Work out the finished part from the listing and answer in its coordinate system (mm). A direction names the side the tool comes from. Coordinates: 2 decimals unless noted, no trailing zeros. Loops run counter-clockwise (first coordinate to the right, second up) from the corner with the lowest first, then second, coordinate; pieces in that order, holes last. Notation, with made-up numbers: (-27.5, -7.5) -> (4.5, -7.5) arc R19 ccw to (4.5, -1.5) -> close; hole circle Ø2 at (72, 1.25). An arc over 180 degrees is marked (long way). Use a Markdown table: item, result. Add a question column.
```python
from build123d import *

# Parameters (mm, degrees)
BOSS_EXTRUDE1_DEPTH = 75
SKETCH4_W           = 56
SKETCH4_H           = 70
CUT_EXTRUDE1_DEPTH  = 36
SKETCH21_R          = 0.875
BOSS_EXTRUDE3_DEPTH = 5
CUT_EXTRUDE2_REACH  = 77
SKETCH23_W          = 11.9
SKETCH23_H          = 2.9
CUT_EXTRUDE3_REACH  = 70.5
SKETCH24_W          = 11
SKETCH24_H          = 3
CUT_EXTRUDE4_REACH  = 70.5
SKETCH25_W          = 7
SKETCH25_H          = 2
CUT_EXTRUDE5_REACH  = 70.5
SKETCH26_W          = 7.2
SKETCH26_H          = 2
CUT_EXTRUDE6_REACH  = 77
SKETCH27_W          = 16
SKETCH27_H          = 2.9
CUT_EXTRUDE7_REACH  = 70.5
SKETCH28_W          = 6
SKETCH28_H          = 9
CUT_EXTRUDE8_REACH  = 70.5
SKETCH29_W          = 21
SKETCH29_H          = 5
CUT_EXTRUDE9_REACH  = 77
SKETCH30_W          = 6
SKETCH30_H          = 8
CUT_EXTRUDE10_REACH = 70.5
SKETCH31_W          = 49
SKETCH31_H          = 7
CUT_EXTRUDE11_REACH = 70.5
SKETCH32_W          = 6
SKETCH32_H          = 7


with BuildPart() as part:
    # Sketch1 → Boss-Extrude1 (new body)
    with BuildSketch(Plane.XY):
        Polygon((-37.771390637, 7.690116692), (-37.771390637, 10.690116692), (38.228609363, 10.690116692), (38.228609363, 7.690116692), (30.728609363, 7.690116692), (30.728609363, -28.309883308), (-30.271390637, -28.309883308), (-30.271390637, 7.690116692), align=None)
    extrude(amount=BOSS_EXTRUDE1_DEPTH)

    # Sketch4 → Cut-Extrude1 (cut)
    with BuildSketch(Plane(origin=(0, 10.690116692, 0), x_dir=(1, 0, 0), z_dir=(0, 1, 0))):
        with Locations((0.228609363, -37.5)):
            Rectangle(SKETCH4_W, SKETCH4_H)
    extrude(amount=-CUT_EXTRUDE1_DEPTH, mode=Mode.SUBTRACT)

    # Sketch21 → Boss-Extrude3 (add)
    with BuildSketch(Plane(origin=(0, -25.309883308, 0), x_dir=(1, 0, 0), z_dir=(0, 1, 0))):
        with Locations((-11.271390637, -8.5)):
            Circle(SKETCH21_R)
        with Locations((11.728609363, -8.5)):
            Circle(SKETCH21_R)
        with Locations((-11.271390637, -66.5)):
            Circle(SKETCH21_R)
        with Locations((11.728609363, -66.5)):
            Circle(SKETCH21_R)
    extrude(amount=BOSS_EXTRUDE3_DEPTH)

    # Sketch23 → Cut-Extrude2 (cut, up to next)
    with BuildSketch(Plane(origin=(0, 0, 0), x_dir=(-1, 0, 0), z_dir=(0, 0, -1)), mode=Mode.PRIVATE) as cut_extrude2_sk1:
        with Locations((-2.078609363, -23.759883308)):
            Rectangle(SKETCH23_W, SKETCH23_H)
    cut_extrude2_tool1 = extrude(cut_extrude2_sk1.sketch, amount=-CUT_EXTRUDE2_REACH, mode=Mode.PRIVATE) & part.part
    add(cut_extrude2_tool1.solids().sort_by_distance((2.078609, -23.759883, 0))[0], mode=Mode.SUBTRACT)

    # Sketch24 → Cut-Extrude3 (cut, up to next)
    with BuildSketch(Plane.ZY.offset(30.271390637), mode=Mode.PRIVATE) as cut_extrude3_sk1:
        with Locations((17.5, -21.809883308)):
            Rectangle(SKETCH24_W, SKETCH24_H)
    cut_extrude3_tool1 = extrude(cut_extrude3_sk1.sketch, amount=-CUT_EXTRUDE3_REACH, mode=Mode.PRIVATE) & part.part
    add(cut_extrude3_tool1.solids().sort_by_distance((-30.271391, -21.809883, 17.5))[0], mode=Mode.SUBTRACT)

    # Sketch25 → Cut-Extrude4 (cut, up to next)
    with BuildSketch(Plane.ZY.offset(30.271390637), mode=Mode.PRIVATE) as cut_extrude4_sk1:
        with Locations((46.4, -22.309883308)):
            Rectangle(SKETCH25_W, SKETCH25_H)
    cut_extrude4_tool1 = extrude(cut_extrude4_sk1.sketch, amount=-CUT_EXTRUDE4_REACH, mode=Mode.PRIVATE) & part.part
    add(cut_extrude4_tool1.solids().sort_by_distance((-30.271391, -22.309883, 46.4))[0], mode=Mode.SUBTRACT)

    # Sketch26 → Cut-Extrude5 (cut, up to next)
    with BuildSketch(Plane.ZY.offset(30.271390637), mode=Mode.PRIVATE) as cut_extrude5_sk1:
        with Locations((59.4, -22.309883308)):
            Rectangle(SKETCH26_W, SKETCH26_H)
    cut_extrude5_tool1 = extrude(cut_extrude5_sk1.sketch, amount=-CUT_EXTRUDE5_REACH, mode=Mode.PRIVATE) & part.part
    add(cut_extrude5_tool1.solids().sort_by_distance((-30.271391, -22.309883, 59.4))[0], mode=Mode.SUBTRACT)

    # Sketch27 → Cut-Extrude6 (cut, up to next)
    with BuildSketch(Plane.XY.offset(75), mode=Mode.PRIVATE) as cut_extrude6_sk1:
        with Locations((0.228609363, -23.759883308)):
            Rectangle(SKETCH27_W, SKETCH27_H)
    cut_extrude6_tool1 = extrude(cut_extrude6_sk1.sketch, amount=-CUT_EXTRUDE6_REACH, mode=Mode.PRIVATE) & part.part
    add(cut_extrude6_tool1.solids().sort_by_distance((0.228609, -23.759883, 75))[0], mode=Mode.SUBTRACT)

    # Sketch28 → Cut-Extrude7 (cut, up to next)
    with BuildSketch(Plane.ZY.offset(30.271390637), mode=Mode.PRIVATE) as cut_extrude7_sk1:
        with Locations((20, -7.809883308)):
            Rectangle(SKETCH28_W, SKETCH28_H)
    cut_extrude7_tool1 = extrude(cut_extrude7_sk1.sketch, amount=-CUT_EXTRUDE7_REACH, mode=Mode.PRIVATE) & part.part
    add(cut_extrude7_tool1.solids().sort_by_distance((-30.271391, -7.809883, 20))[0], mode=Mode.SUBTRACT)

    # Sketch29 → Cut-Extrude8 (cut, up to next)
    with BuildSketch(Plane.ZY.offset(30.271390637), mode=Mode.PRIVATE) as cut_extrude8_sk1:
        with Locations((38.5, -9.809883308)):
            Rectangle(SKETCH29_W, SKETCH29_H)
    cut_extrude8_tool1 = extrude(cut_extrude8_sk1.sketch, amount=-CUT_EXTRUDE8_REACH, mode=Mode.PRIVATE) & part.part
    add(cut_extrude8_tool1.solids().sort_by_distance((-30.271391, -9.809883, 38.5))[0], mode=Mode.SUBTRACT)

    # Sketch30 → Cut-Extrude9 (cut, up to next)
    with BuildSketch(Plane(origin=(0, 0, 0), x_dir=(-1, 0, 0), z_dir=(0, 0, -1)), mode=Mode.PRIVATE) as cut_extrude9_sk1:
        with Locations((9.771390637, -6.309883308)):
            Rectangle(SKETCH30_W, SKETCH30_H)
    cut_extrude9_tool1 = extrude(cut_extrude9_sk1.sketch, amount=-CUT_EXTRUDE9_REACH, mode=Mode.PRIVATE) & part.part
    add(cut_extrude9_tool1.solids().sort_by_distance((-9.771391, -6.309883, 0))[0], mode=Mode.SUBTRACT)

    # Sketch31 → Cut-Extrude10 (cut, up to next)
    with BuildSketch(Plane(origin=(30.728609363, 0, 0), x_dir=(0, 0, -1), z_dir=(1, 0, 0)), mode=Mode.PRIVATE) as cut_extrude10_sk1:
        with Locations((-37.5, 3.190116692)):
            Rectangle(SKETCH31_W, SKETCH31_H)
    cut_extrude10_tool1 = extrude(cut_extrude10_sk1.sketch, amount=-CUT_EXTRUDE10_REACH, mode=Mode.PRIVATE) & part.part
    add(cut_extrude10_tool1.solids().sort_by_distance((30.728609, 3.190117, 37.5))[0], mode=Mode.SUBTRACT)

    # Sketch32 → Cut-Extrude11 (cut, up to next)
    with BuildSketch(Plane.ZY.offset(30.271390637), mode=Mode.PRIVATE) as cut_extrude11_sk1:
        with Locations((53, 3.190116692)):
            Rectangle(SKETCH32_W, SKETCH32_H)
    cut_extrude11_tool1 = extrude(cut_extrude11_sk1.sketch, amount=-CUT_EXTRUDE11_REACH, mode=Mode.PRIVATE) & part.part
    add(cut_extrude11_tool1.solids().sort_by_distance((-30.271391, 3.190117, 53))[0], mode=Mode.SUBTRACT)


solid = part.part
```
Item 1: Find the intervals of material crossed by probe 1 along Z at (x, y) = (11, -4); probe 2 along X at (y, z) = (-21, 40); probe 3 along X at (y, z) = (8.5, 52.5), in increasing order.
Item 2: Section D-D (z = 69) is taken. Determine the outline of the cut face in (x, y).
Item 3: Given pin 1 (2 mm diameter, centred on y = -24.5, z = 73.5, fed in from -X); pin 2 (0.8 mm diameter, centred on y = -23.5, z = 1.5, fed in from +X); pin 3 (6 mm diameter, centred on x = 35.5, z = 23, fed in from -Y), each flat-ended and moving along its own axis, determine where each tip first touches the part or whether it passes through.
Item 4: Section B-B (x = 1.5) is taken. Determine the outline of the cut face in (y, z).
Item 5: Section A-A (z = 20.5) is taken. Determine the outline of the cut face in (x, y), then the cut area to 4 significant figures.
Item 6: Section C-C (y = -15.5) is taken. Determine the outline of the cut face in (x, z).
Item 7: For faces 5 (the face through (-10, -10.31, 1)), 6 (the face through (-29, -10, 28)), 7 (the face through (8.029, -24, 1)), determine the directions among +Z, -Z, +X, -X, +Y, -Y from which every point of the face is accessible in a straight line to the end or side of a thin tool.
Item 8: For a pull along Y with two mould halves and no side action, classify faces 1 (the face through (-28, 10.69, 37)), 2 (the face through (-7.771, -24, 74)), 3 (the face through (1, -9, 75)), 4 (the face through (-29, 3, 56)) as +Y half, -Y half, draft (parallel to the pull), parting line (faces both ways), or undercut.
Output:
| question | item | result |
|---|---|---|
| 1 | probe 1 | z = 0 to 2.5, 72.5 to 75 |
| 1 | probe 2 | x = -30.27 to -27.77, 28.23 to 30.73 |
| 1 | probe 3 | x = -37.77 to -27.77, 28.23 to 38.23 |
| 2 | outline | (-37.77, 7.69) -> (-30.27, 7.69) -> (-30.27, -28.31) -> (30.73, -28.31) -> (30.73, 7.69) -> (38.23, 7.69) -> (38.23, 10.69) -> (28.23, 10.69) -> (28.23, -25.31) -> (-27.77, -25.31) -> (-27.77, 10.69) -> (-37.77, 10.69) -> close |
| 3 | pin 1 | stops at x = -30.27 |
| 3 | pin 2 | stops at x = 30.73 |
| 3 | pin 3 | stops at y = 7.69 |
| 4 | outline | (-28.31, 0) -> (-25.21, 0) -> (-25.21, 2.5) -> (-25.31, 2.5) -> (-25.31, 72.5) -> (-25.21, 72.5) -> (-25.21, 75) -> (-28.31, 75) -> close; (-22.31, 0) -> (10.69, 0) -> (10.69, 2.5) -> (-22.31, 2.5) -> close; (-22.31, 72.5) -> (10.69, 72.5) -> (10.69, 75) -> (-22.31, 75) -> close |
| 5 | outline | (-37.77, 7.69) -> (-30.27, 7.69) -> (-30.27, -3.31) -> (-27.77, -3.31) -> (-27.77, 10.69) -> (-37.77, 10.69) -> close; (-30.27, -28.31) -> (30.73, -28.31) -> (30.73, -0.31) -> (28.23, -0.31) -> (28.23, -25.31) -> (-27.77, -25.31) -> (-27.77, -23.31) -> (-30.27, -23.31) -> close; (-30.27, -20.31) -> (-27.77, -20.31) -> (-27.77, -12.31) -> (-30.27, -12.31) -> close; (28.23, 6.69) -> (30.73, 6.69) -> (30.73, 7.69) -> (38.23, 7.69) -> (38.23, 10.69) -> (28.23, 10.69) -> close |
| 5 | area | 360.5 mm2 |
| 6 | outline | (-30.27, 0) -> (30.73, 0) -> (30.73, 75) -> (-30.27, 75) -> close; hole (-27.77, 2.5) -> (28.23, 2.5) -> (28.23, 72.5) -> (-27.77, 72.5) -> close |
| 7 | face 5 | -Z |
| 7 | face 6 | -X |
| 7 | face 7 | +Z, -Z |
| 8 | face 1 | +Y half |
| 8 | face 2 | undercut |
| 8 | face 3 | draft |
| 8 | face 4 | undercut |
